```python
from build123d import *

# Parameters (mm, degrees)
SKETCH1_W           = 287
SKETCH1_H           = 290
BOSS_EXTRUDE1_DEPTH = 7.5
CHAMFER1_SIZE       = 10
SKETCH3_R           = 8
CUT_EXTRUDE1_DEPTH  = 16


with BuildPart() as part:
    # Sketch1 → Boss-Extrude1 (new body, symmetric)
    with BuildSketch(Plane(origin=(0, 0, 0), x_dir=(1, 0, 0), z_dir=(0, 1, 0))):
        with Locations((143.5, 145)):
            Rectangle(SKETCH1_W, SKETCH1_H)
    extrude(amount=BOSS_EXTRUDE1_DEPTH, both=True)

    # Chamfer1
    chamfer1_edges = [part.edges().sort_by_distance(p)[0] for p in [
        (0, 0, -290),
        (287, 0, -290),
        (287, 0, 0),
        (0, 0, 0),
    ]]
    chamfer(chamfer1_edges, length=CHAMFER1_SIZE)

    # Sketch3 → Cut-Extrude1 (cut)
    with BuildSketch(Plane(origin=(0, 7.5, 0), x_dir=(1, 0, 0), z_dir=(0, 1, 0))):
        with Locations((40, 35)):
            Circle(SKETCH3_R)
        with Locations((40, 250)):
            Circle(SKETCH3_R)
        with Locations((247, 250)):
            Circle(SKETCH3_R)
        with Locations((247, 35)):
            Circle(SKETCH3_R)
    extrude(amount=-CUT_EXTRUDE1_DEPTH, mode=Mode.SUBTRACT)


solid = part.part
```
Check sheet for the modelled part. Datum: model origin and axes. Units: mm. Give positions to 0.01 mm unless a question says otherwise; leave off trailing zeros. Order: outer loops, then holes, each group sorted by start corner. A loop starts at its lowest first (then second) coordinate and runs counter-clockwise, first axis right, second up. Notation, with made-up numbers: (-39.75, -6.5) -> (-13.75, -6.5) arc R34 ccw to (-13.75, 30.5) -> close; hole circle Ø5 at (52, -39). An arc over 180 degrees is marked (long way). Return JSON: item names as keys, results as strings.
1. Cross-section at B-B, the plane x = 247. Record the cut outline in (y, z).
From the geometry:
{"outline": "(-7.5, -290) -> (7.5, -290) -> (7.5, -258) -> (-7.5, -258) -> close; (-7.5, -242) -> (7.5, -242) -> (7.5, -43) -> (-7.5, -43) -> close; (-7.5, -27) -> (7.5, -27) -> (7.5, 0) -> (-7.5, 0) -> close"}
2. Material ranges on probe 1 along X at (y, z) = (0, -35); probe 2 along X at (y, z) = (-5.5, -28), recorded low to high. Write a range as [from, to].
From the geometry:
{"probe 1": "[0, 32], [48, 239], [255, 287]", "probe 2": "[0, 36.13], [43.87, 243.13], [250.87, 287]"}
3. Cross-section at A-A, the plane z = -35. Record the cut outline in (x, y), plus the area to 4 significant figures.
From the geometry:
{"outline": "(0, -7.5) -> (32, -7.5) -> (32, 7.5) -> (0, 7.5) -> close; (48, -7.5) -> (239, -7.5) -> (239, 7.5) -> (48, 7.5) -> close; (255, -7.5) -> (287, -7.5) -> (287, 7.5) -> (255, 7.5) -> close", "area": "3,825 mm^2"}
4. Mould release check, pull along X, two halves, no side actions. Record for faces 1 (the cylindrical face through (38.959, 0.105, -42.932)), 2 (the flat face through (282, 0, -5)), 3 (the cylindrical face through (241.1, 0.1, -40.4)), 4 (the flat face through (141, -7.5, -147)): +X half, -X half, draft (parallel to the pull), parting line (faces both ways), or undercut.
From the geometry:
{"face 1": "undercut", "face 2": "+X half", "face 3": "undercut", "face 4": "draft"}
